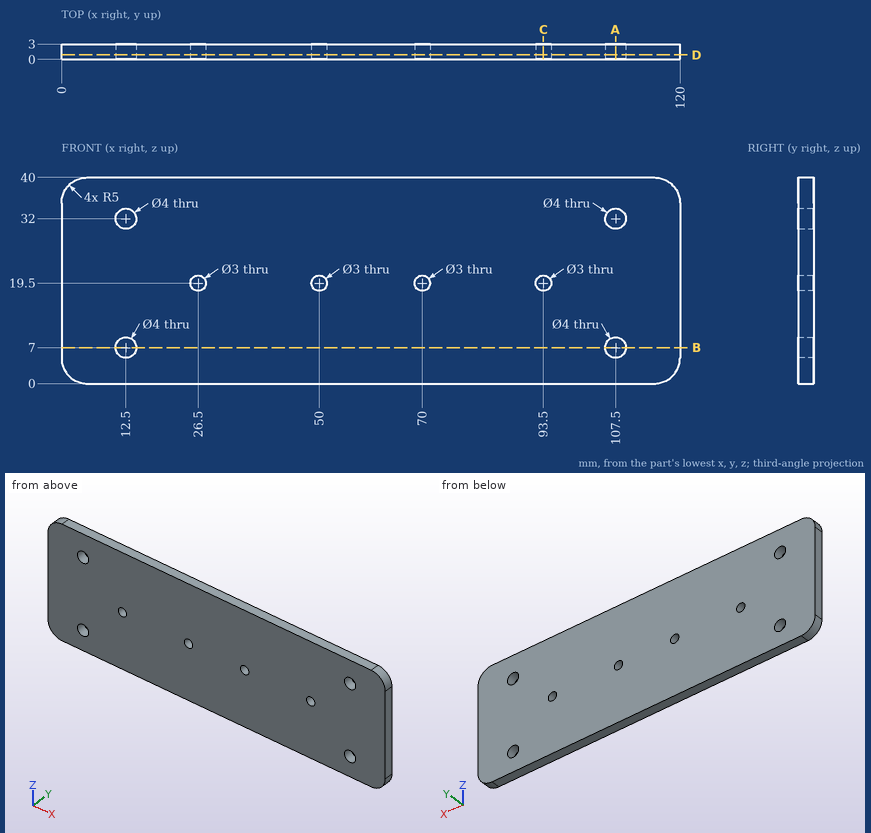
Can you work these out from the drawing? Everything is in mm from the part's minimum corner. Round coordinates to 2 decimals unless told otherwise and drop trailing zeros. Loops run counter-clockwise (first coordinate to the right, second up) from the corner with the lowest first, then second, coordinate; pieces in that order, holes last. Notation, with made-up numbers: M 63,59.5 L 108,59.5 A31 cw 108,88.5 Z; hole C 57.25,41.25 d7. An arc over 180 degrees is marked long. Answer in a Markdown table with one row per item.
1. Please list where these lines run through material, in increasing order: line 1 (X direction, y = 1.8, z = 19.5); line 2 (X direction, y = 1.6, z = 32); line 3 (Z direction, x = 70, y = 2). Write a range as from..to.
Established:
| item | result |
|---|---|
| line 1 | 0..25, 28..48.5, 51.5..68.5, 71.5..92, 95..120 |
| line 2 | 0..10.5, 14.5..105.5, 109.5..120 |
| line 3 | 0..18, 21..40 |
2. If we section it at A-A, the plane x = 107.5: Please give me the cut outline in (y, z), plus the area to 3 significant figures.
Established:
| item | result |
|---|---|
| outline | M 0,0 L 3,0 L 3,5 L 0,5 Z; M 0,9 L 3,9 L 3,30 L 0,30 Z; M 0,34 L 3,34 L 3,40 L 0,40 Z |
| area | 96.0 mm² |
3. I'm going to push flat-ended pins straight in: pin 1 Ø1 at (y, z) = (1.5, 36) entering from +X; pin 2 Ø1.5 at (x, y) = (29.5, 1.5) entering from -Z. Where does each tip first touch, or does it pass through?
Established:
| item | result |
|---|---|
| pin 1 | x = 119.97 |
| pin 2 | z = 0 |
4. If we section it at C-C, the plane x = 93.5: Please give me the cut outline in (y, z).
Established:
| item | result |
|---|---|
| outline | M 0,0 L 3,0 L 3,18 L 0,18 Z; M 0,21 L 3,21 L 3,40 L 0,40 Z |
5. If we section it at B-B, the plane z = 7: Please give me the cut outline in (x, y), plus the area to 3 significant figures.
Established:
| item | result |
|---|---|
| outline | M 0,0 L 10.5,0 L 10.5,3 L 0,3 Z; M 14.5,0 L 105.5,0 L 105.5,3 L 14.5,3 Z; M 109.5,0 L 120,0 L 120,3 L 109.5,3 Z |
| area | 336 mm² |
6. If we section it at D-D, the plane y = 0.9: Give the number of separate pieces and of enclosed holes in the cut face, plus the area to 3 significant figures.
Established:
| item | result |
|---|---|
| separate pieces | 1 |
| enclosed holes | 8 |
| area | 4,700 mm² |
